Geometry check sheet. Reference: drawing and pictorial views, mm from the part's lowest x, y, z. Round coordinates to 2 decimals unless told otherwise and drop trailing zeros. Order: outer loops, then holes, each group sorted by start corner. A loop starts at its lowest first (then second) coordinate and runs counter-clockwise, first axis right, second up.
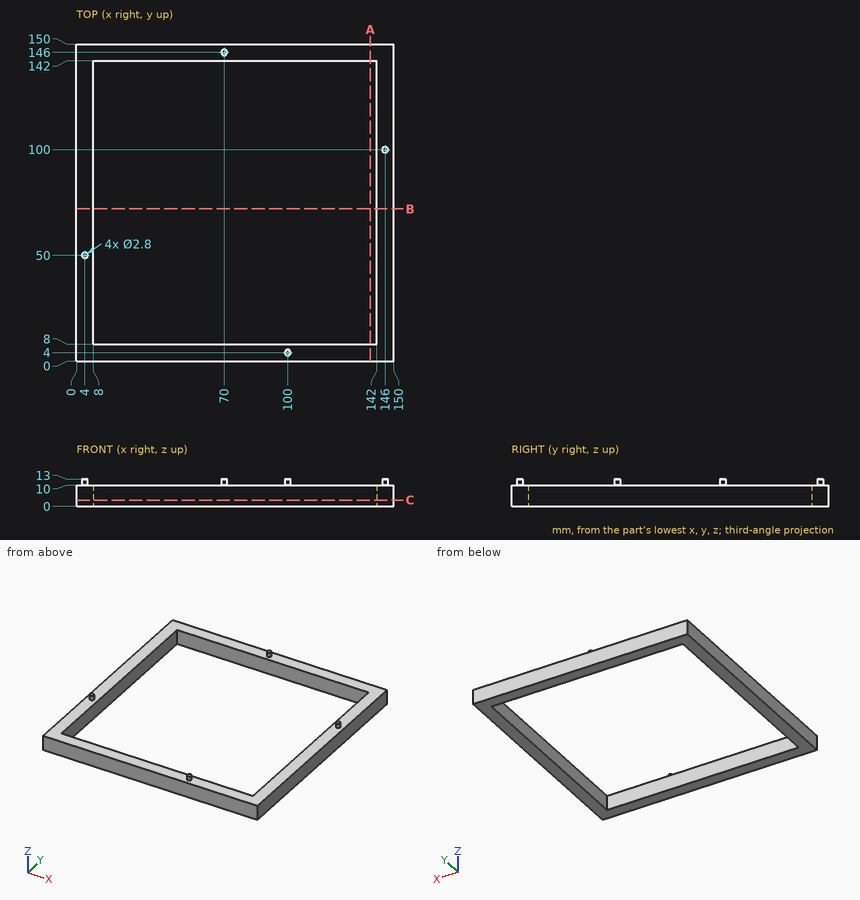
1) Sectioned sample at A-A on x = 139. Record the cut outline in (y, z).
2) Scan line: probe 1 along X at (y, z) = (83.5, 6). Record every from-to range of solid material in increasing order.
3) Sectioned sample at C-C on z = 3. Record the cut outline in (x, y).
4) Go/stop test with a flat-tipped pin: pin 1 Ø2 at (x, z) = (125, 2.5) entering from -Y. Record where the tip stops, or that it passes through.
Returned:
1. outline: (0, 0) - (8, 0) - (8, 10) - (0, 10) - close; (142, 0) - (150, 0) - (150, 10) - (142, 10) - close
2. probe 1: x = 0 to 8, 142 to 150
3. outline: (0, 0) - (150, 0) - (150, 150) - (0, 150) - close; hole (8, 8) - (142, 8) - (142, 142) - (8, 142) - close
4. pin 1: stops at y = 0
